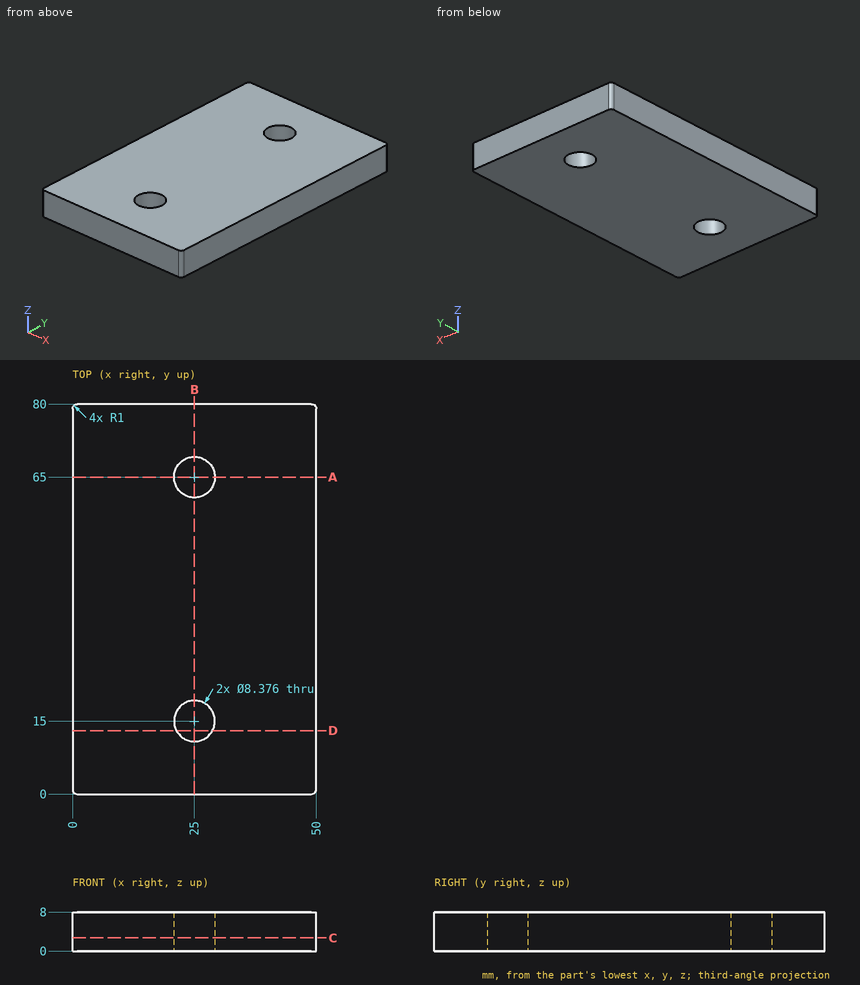
Here's the drawing with two shaded views (mm, measured from the low corner). I have some questions. Give positions to 0.01 mm unless a question says otherwise; leave off trailing zeros. Loops run counter-clockwise (first coordinate to the right, second up) from the corner with the lowest first, then second, coordinate; pieces in that order, holes last. Notation, with made-up numbers: (66.5, -22) - (125.5, -22) arc R9 cw to (125.5, -9) - close; hole circle Ø11 at (41, 40). An arc over 180 degrees is marked (long way). Return JSON: item names as keys, results as strings.
1. I'm going to push flat-ended pins straight in: pin 1 Ø6 at (x, y) = (32.5, 51.5) entering from -Z; pin 2 Ø7.5 at (x, y) = (25, 15) entering from +Z. Where does each tip first touch, or does it pass through?
Output values:
{"pin 1": "stops at z = 0", "pin 2": "passes through"}
2. If I drill on line 1 (Y direction, x = 25, z = 4.75); line 2 (X direction, y = 65, z = 2.25); line 3 (Y direction, x = 23.5, z = 6.25), over which ranges is the centre line in solid material (lowest first)?
Output values:
{"line 1": "y = 0 to 10.81, 19.19 to 60.81, 69.19 to 80", "line 2": "x = 0 to 20.81, 29.19 to 50", "line 3": "y = 0 to 11.09, 18.91 to 61.09, 68.91 to 80"}
3. I want a section at D-D on y = 13. Please give me the cut outline in (x, z).
Output values:
{"outline": "(0, 0) - (21.32, 0) - (21.32, 8) - (0, 8) - close; (28.68, 0) - (50, 0) - (50, 8) - (28.68, 8) - close"}
4. I want a section at C-C on z = 2.75. Please give me the cut outline in (x, y).
Output values:
{"outline": "(0, 1) arc R1 ccw to (1, 0) - (49, 0) arc R1 ccw to (50, 1) - (50, 79) arc R1 ccw to (49, 80) - (1, 80) arc R1 ccw to (0, 79) - close; hole circle Ø8.38 at (25, 15); hole circle Ø8.38 at (25, 65)"}
5. I want a section at A-A on y = 65. Please give me the cut outline in (x, z), and give its area (3 significant figures).
Output values:
{"outline": "(0, 0) - (20.81, 0) - (20.81, 8) - (0, 8) - close; (29.19, 0) - (50, 0) - (50, 8) - (29.19, 8) - close", "area": "333 mm²"}
6. I want a section at B-B on x = 25. Please give me the cut outline in (y, z).
Output values:
{"outline": "(0, 0) - (10.81, 0) - (10.81, 8) - (0, 8) - close; (19.19, 0) - (60.81, 0) - (60.81, 8) - (19.19, 8) - close; (69.19, 0) - (80, 0) - (80, 8) - (69.19, 8) - close"}
